Verification items for the finished model (mm, model axes). A direction names the side the tool comes from. Round coordinates to 2 decimals unless told otherwise and drop trailing zeros. Write each loop counter-clockwise with the first axis right and the second up, starting at its lowest first coordinate (ties: lowest second). Pieces come first, ordered by that corner, then holes. Notation, with made-up numbers: (86, 53) - (119, 53) arc R24 cw to (119, 81) - close; hole circle Ø8 at (-10, 17.5). An arc over 180 degrees is marked (long way). Answer as a JSON object with one key per item and string values. Group by question number.
1) Section check B-B (x = 20). Enter the section's corners in (y, z), then the cut area to 3 significant figures.
2) Section check D-D (y = 27). Enter the section's corners in (x, z), then the cut area to 3 significant figures.
3) Mould release check, pull along X, two halves, no side actions. Record for faces 1 (the flat face through (-30.39, 8.76, 2.99)), 2 (the flat face through (50, 0, 1)), 3 (the flat face through (0, 49, 3)): +X half, -X half, draft (parallel to the pull), parting line (faces both ways), or undercut.
4) Section check C-C (z = 0.95). State how many separate pieces and enclosed holes the cut face has, then the cut area to 3 significant figures.
5) Thickness scan on line 1 (Y direction, x = 0, z = 0.8); line 2 (X direction, y = 28.5, z = 0.65); line 3 (X direction, y = 13, z = 2.7). Record the ranges inside material, lowest first.
6) Set-up check for faces 4 (the flat face through (11.24, 1.16, 2.99)), 5 (the flat face through (30.62, 8.76, 2.99)), 6 (the flat face through (30, 9.75, 1)): record each of +Z, -Z, +X, -X, +Y, -Y from which the full face is reachable in a straight line by a thin tool's end or side.
7) Go/stop test with flat-tipped pins: pin 1 Ø1.6 at (x, z) = (29.5, 0.5) entering from +Y; pin 2 Ø0.6 at (y, z) = (28, 1) entering from -X; pin 3 Ø3 at (x, y) = (1, 38.5) entering from +Z. Record where each tip stops, or that it passes through.
8) Section check A-A (y = 20). Enter the section's corners in (x, z), then the cut area to 3 significant figures.
```python
from build123d import *

# Parameters (mm, degrees)
F0_R     = 1.75
F1_DEPTH = 4
F2_SIZE  = 1.75
F3_SIZE  = 2


with BuildPart() as f1:
    # F0 (on Top) → F1 (new body)
    with BuildSketch(Plane.XY):
        Polygon((10.25, 10.25), (10.25, -10.25), (50, -10.25), (50, 9.75), (10, 50), (0, 50), (-10, 50), (-50, 9.75), (-50, -10.25), (-10.25, -10.25), (-10.25, 10.25), (0, 10.25), align=None)
        with Locations((-40, 0)):
            Circle(F0_R, mode=Mode.SUBTRACT)
        with Locations((-20, 0)):
            Circle(F0_R, mode=Mode.SUBTRACT)
        with Locations((20, 0)):
            Circle(F0_R, mode=Mode.SUBTRACT)
        with Locations((40, 0)):
            Circle(F0_R, mode=Mode.SUBTRACT)
        Polygon((-35.901716, 9.75), (-10, 35.813601), (-10, 24.687961), (-24.845179, 9.75), align=None, mode=Mode.SUBTRACT)
        with Locations((0, 20)):
            Circle(F0_R, mode=Mode.SUBTRACT)
        Polygon((10, 24.687961), (10, 35.813601), (35.901716, 9.75), (24.845179, 9.75), align=None, mode=Mode.SUBTRACT)
        with Locations((0, 40)):
            Circle(F0_R, mode=Mode.SUBTRACT)
    extrude(amount=F1_DEPTH)

    # F2
    f2_edges = [f1.edges().sort_by_distance(p)[0] for p in [
        (-21.75, 0, 4),
        (-41.75, 0, 4),
        (-1.75, 20, 4),
        (-1.75, 40, 4),
        (18.25, 0, 4),
        (38.25, 0, 4),
    ]]
    chamfer(f2_edges, length=F2_SIZE)

    # F3
    f3_edges = [f1.edges().sort_by_distance(p)[0] for p in [
        (-30, 29.875, 4),
        (-50, -0.25, 4),
        (-30.125, -10.25, 4),
        (-10.25, 0, 4),
        (0, 10.25, 4),
        (10.25, 0, 4),
        (30.125, -10.25, 4),
        (50, -0.25, 4),
        (30, 29.875, 4),
        (0, 50, 4),
        (22.950858, 22.781801, 4),
        (10, 30.250781, 4),
        (17.422589, 17.218981, 4),
        (30.373447, 9.75, 4),
        (-17.422589, 17.218981, 4),
        (-30.373447, 9.75, 4),
        (-22.950858, 22.781801, 4),
        (-10, 30.250781, 4),
    ]]
    chamfer(f3_edges, length=F3_SIZE)


solid = f1.part
```
Returned:
{
 "1": {"outline": "(-10.25, 0) - (-1.75, 0) - (-1.75, 2.25) - (-3.5, 4) - (-8.25, 4) - (-10.25, 2) - close; (1.75, 0) - (14.63, 0) - (14.63, 2) - (11.79, 4) - (3.5, 4) - (1.75, 2.25) - close; (25.75, 0) - (39.94, 0) - (39.94, 2) - (37.1, 4) - (28.59, 4) - (25.75, 2) - close", "area": "129 mm2"},
 "2": {"outline": "(-32.86, 0) - (-18.76, 0) - (-18.76, 2) - (-21.58, 4) - (-30.04, 4) - (-32.86, 2) - close; (-10, 0) - (10, 0) - (10, 2) - (8, 4) - (-8, 4) - (-10, 2) - close; (18.76, 0) - (32.86, 0) - (32.86, 2) - (30.04, 4) - (21.58, 4) - (18.76, 2) - close", "area": "178 mm2"},
 "3": {"face 1": "undercut", "face 2": "+X half", "face 3": "draft"},
 "4": {"separate pieces": "1", "enclosed holes": "8", "area": "3,480 mm2"},
 "5": {"line 1": "10.25 to 18.25, 21.75 to 38.25, 41.75 to 50", "line 2": "-31.37 to -17.27, -10 to 10, 17.27 to 31.37", "line 3": "-45.78 to -33.66, -20.63 to 20.63, 33.66 to 45.78"},
 "6": {"face 4": "+Z, -Y", "face 5": "+Z", "face 6": "+Z, -Z"},
 "7": {"pin 1": "y = 31.18", "pin 2": "x = -32.16", "pin 3": "z = 3.8"},
 "8": {"outline": "(-39.81, 0) - (-25.72, 0) - (-25.72, 2) - (-28.54, 4) - (-36.99, 4) - (-39.81, 2) - close; (-14.66, 0) - (-1.75, 0) - (-1.75, 2.25) - (-3.5, 4) - (-11.84, 4) - (-14.66, 2) - close; (1.75, 0) - (14.66, 0) - (14.66, 2) - (11.84, 4) - (3.5, 4) - (1.75, 2.25) - close; (25.72, 0) - (39.81, 0) - (39.81, 2) - (36.99, 4) - (28.54, 4) - (25.72, 2) - close", "area": "196 mm2"}
}
